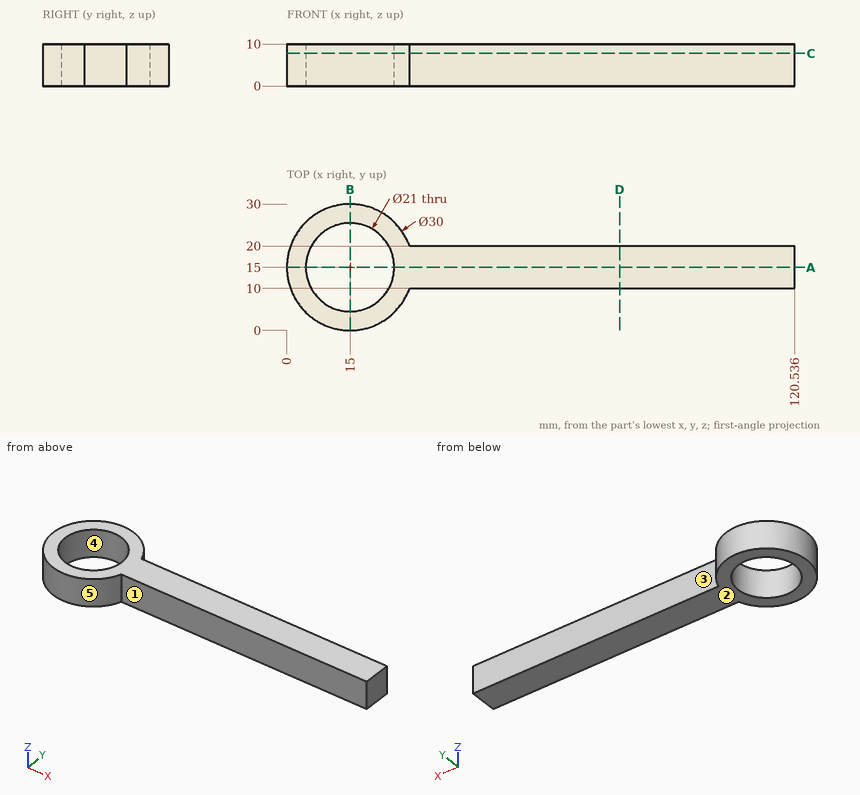
Answer from the drawing. Dimensions are ordinates in mm from the lowest x, y and z of the part. A direction names the side the tool comes from. Coordinates: 2 decimals unless noted, no trailing zeros. Loops run counter-clockwise (first coordinate to the right, second up) from the corner with the lowest first, then second, coordinate; pieces in that order, holes last.
Q1. The part is cut by section C-C on z = 7.75. Write down the section's boundary in (x, y) (1 decimal).
Q2. The part is cut by section A-A on y = 15. Write down the section's boundary in (x, z) (1 decimal).
Q3. Each of these flat-tipped pins is pushed along its axis until it touches: pin 1 Ø2 at (x, z) = (102.5, 7.5) entering from +Y; pin 2 Ø3 at (y, z) = (18.5, 3.5) entering from -X; pin 3 Ø1 at (y, z) = (25.5, 9) entering from +X. Where does it stop, or does it pass through?
Q4. Consider probe 1 along Y at (x, z) = (15, 7); probe 2 along Y at (x, z) = (65.5, 3.5); probe 3 along Y at (x, z) = (21.5, 6.75) (1 decimal). Determine where each line is inside the solid, lowest interval first.
Q5. Which of the six approach directions +Z, -Z, +X, -X, +Y, -Y give full straight-line access (tool end or side, diameter ignored) to the marked faces 1 and 2?
Q6. The part is cut by section B-B on x = 15. Write down the section's boundary in (y, z).
Q7. The part is cut by section D-D on x = 79. Write down the section's boundary in (y, z), and give its area (3 significant figures).
Q8. The mould has two halves that part along X. Classify the marked faces 3, 4 and 5: +X half, -X half, draft (parallel to the pull), parting line (faces both ways), or undercut.
Results below:
1. outline: (29.1, 10) - (120.5, 10) - (120.5, 20) - (29.1, 20) arc R15 ccw (long way) to start; hole circle Ø21 at (15, 15)
2. outline: (0, 0) - (4.5, 0) - (4.5, 10) - (0, 10) - close; (25.5, 0) - (120.5, 0) - (120.5, 10) - (25.5, 10) - close
3. pin 1: stops at y = 20
3. pin 2: stops at x = 0.13
3. pin 3: stops at x = 26.18
4. probe 1: y = 0 to 4.5, 25.5 to 30
4. probe 2: y = 10 to 20
4. probe 3: y = 1.5 to 6.8, 23.2 to 28.5
5. face 1: +Z, -Z, +X, -Y
5. face 2: -Z, +X, -X, +Y, -Y
6. outline: (0, 0) - (4.5, 0) - (4.5, 10) - (0, 10) - close; (25.5, 0) - (30, 0) - (30, 10) - (25.5, 10) - close
7. outline: (10, 0) - (20, 0) - (20, 10) - (10, 10) - close
7. area: 100 mm2
8. face 3: draft
8. face 4: undercut
8. face 5: parting line
